Autodesk Fusion 360 part; units mm, degrees
sketch "Sketch1" plane through (0, 0, 0) normal (0, 1, 0) x (1, 0, 0)
  circle A0 centre (0, 0) radius 5.5
  dimension "d1" = 11
ref_plane "WorkPlane1" through (0, 20, 0) normal (0, 1, 0) x (1, 0, 0)
sketch "Sketch2" plane through (0, 20, 0) normal (0, 1, 0) x (1, 0, 0)
  circle A0 centre (0, 0) radius 5.5
  dimension "d3" = 11
ref_plane "WorkPlane2" through (0, -2, 0) normal (0, 1, 0) x (1, 0, 0)
sketch "Sketch3" plane through (0, -2, 0) normal (0, 1, 0) x (1, 0, 0)
  circle A0 centre (0, 0) radius 4.5
  dimension "d5" = 9
ref_plane "WorkPlane3" through (0, -5, 0) normal (0, 1, 0) x (1, 0, 0)
sketch "Sketch4" plane through (0, -5, 0) normal (0, 1, 0) x (1, 0, 0)
  circle A0 centre (0, 0) radius 4.5
  dimension "d7" = 9
ref_plane "WorkPlane4" through (0, -16, 0) normal (0, 1, 0) x (1, 0, 0)
sketch "Sketch5" plane through (0, -16, 0) normal (0, 1, 0) x (1, 0, 0)
  circle A0 centre (0, 0) radius 3.5
  dimension "d9" = 7
loft "Loft1" add profiles "Sketch2", "Sketch1" section 1 section 2 makes body 1
loft "Loft2" add profiles "Sketch3" section 1 face at (-1.4907, 0, -0.2732) section 2 on bodies 1 bodies 1
loft "Loft3" add profiles "Sketch4" section 1 face at (0.9352, -2, -1.1727) section 2 on bodies 1 bodies 1
loft "Loft4" add profiles "Sketch5" section 1 face at (0.9352, -5, -1.1727) section 2 on bodies 1 bodies 1
sketch "Sketch6" plane through (0, 0, 0) normal (1, 0, 0) x (0, 1, 0)
  line L0 (-10.5, 5.5424) -> (-10.5, -7.5313)
  line L1 (-5, 0.5) -> (-16, 0.5)
  line L2 (-16, 0.5) -> (-16, -0.5)
  line L3 (-16, -0.5) -> (-5, -0.5)
  line L4 (-5, -0.5) -> (-5, 0.5)
  line L5 (-5, 0.5) -> (-16, -0.5) construction
  line L6 (-16, 0.5) -> (-5, -0.5) construction
  line L7 (-14, 5) -> (-13, 5)
  line L8 (-13, 5) -> (-13, -5)
  line L9 (-13, -5) -> (-14, -5)
  line L10 (-14, -5) -> (-14, 5)
  line L11 (-11, 5) -> (-10, 5)
  line L12 (-10, 5) -> (-10, -5)
  line L13 (-10, -5) -> (-11, -5)
  line L14 (-11, -5) -> (-11, 5)
  line L15 (-8, 5) -> (-7, 5)
  line L16 (-7, 5) -> (-7, -5)
  line L17 (-7, -5) -> (-8, -5)
  line L18 (-8, -5) -> (-8, 5)
  point P0 (-10.5, 0)
  point P1 (-10.5, 0)
  dimension "d10" = 11
  dimension "d11" = 1
extrude "Extrude1" cut sketch "Sketch6" along normal blind 5 and the other way blind 5 contours L0 L1 L11 L12 | L0 L1 L11 L14 | L0 L3 L12 L13 | L0 L3 L13 L14 | L1 L15 L16 L18 | L1 L7 L8 L10 | L3 L8 L9 L10 | L3 L16 L17 L18 bodies 1
sketch "Sketch7" plane through (0, -16, 0) normal (0, -1, 0) x (1, 0, 0)
  circle A0 centre (0, 0) radius 3.5
  circle A1 centre (0, 0) radius 1.75
  dimension "d16" = 3.5
extrude "Extrude2" add sketch "Sketch7" against normal blind 11 contours A1 bodies 1
sketch "Sketch8" plane through (0, 20, 0) normal (0, 1, 0) x (-1, 0, 0)
  circle A0 centre (0, 0) radius 5.5
  circle A1 centre (0, 0) radius 4
  dimension "d19" = 8
extrude "Extrude3" cut sketch "Sketch8" against normal blind 1 contours A1 bodies 1
sketch "Sketch9" plane through (0, 19, 0) normal (0, 1, 0) x (-1, 0, 0)
  circle A0 centre (0, 0) radius 4
  circle A1 centre (0, 0) radius 3
  circle A2 centre (0, 0) radius 3.4
  dimension "d22" = 6
  dimension "d23" = 6.8
extrude "Extrude4" cut sketch "Sketch9" against normal blind 10 bodies 1
sketch "Sketch10" plane through (0, 9, 0) normal (0, 1, 0) x (-1, 0, 0)
  circle A0 centre (0, 0) radius 3
  circle A1 centre (0, 0) radius 1
  dimension "d26" = 2
extrude "Extrude5" add sketch "Sketch10" along normal blind 9 contours A1 bodies 1
fillet "Fillet1" radius 0.8 1 edges at (0.9323, 18, -0.3616) on bodies 1
extrude "Extrude6" add sketch "Sketch7" along normal blind 10 contours A1 bodies 1
copy_body "Body->Comp1" bodies 1 removing the originals makes body 2 in component "Component"
sketch "Sketch11" plane through (0, 0, 0) normal (0, 0, 1) x (1, 0, 0)
  line L0 (10, 20) -> (43, 20)
  line L1 (43, 20) -> (43, -16)
  line L2 (43, -16) -> (10, -16)
  line L3 (10, -16) -> (10, 20)
component "Component" placed x (1, 0, 0) y (0, 1, 0) z (0, 0, 1) at (0, 0, 0)
Can you work these out from the model? Positions are in its coordinate system, mm. A direction names the side the tool comes from. Give positions to 0.01 mm unless a question says otherwise; leave off trailing zeros. Order: outer loops, then holes, each group sorted by start corner. A loop starts at its lowest first (then second) coordinate and runs counter-clockwise, first axis right, second up. Notation, with made-up numbers: M 13,-23.75 L 54,-23.75 A17 cw 54,5.25 Z; hole C -39.5,13.25 d7. An arc over 180 degrees is marked long. Use a Markdown table: item, result. Add a question column.
Item 1: Will these pins go through, and if not, where does the flat tip stop? pin 1 (0.5 mm diameter, centred on x = 3, y = -10.5, fed in from -Z); pin 2 (3 mm diameter, centred on x = 0.5, z = 3, fed in from -Y); pin 3 (3 mm diameter, centred on x = 0.5, y = -9.5, fed in from +Z); pin 4 (3 mm diameter, centred on x = -1, z = -1, fed in from +Y).
Item 2: We'd pull the mould along X, two halves only. Please class faces 1 (the flat face through (0, -14, -2)), 2 (the cylindrical face through (0.867, 14.577, -3.905)), 3 (the conical face through (-3.89, -11.65, -0.17)): +X half, -X half, draft (parallel to the pull), parting line (faces both ways), or undercut.
Item 3: For faces 4 (the flat face through (-2, -16, -1)), 5 (the cylindrical face through (3, 14, 0)), 6 (the flat face through (0, -7, -2)), 7 (the flat face through (3, -7.5, 0.5)), which set-ups out of +Z, -Z, +X, -X, +Y, -Y let a thin tool reach every point of the face, with its end or its side?
Item 4: If I drill on L1, parallel to Z at x = 0, y = 11; L2, parallel to Y at x = 1.5, z = 1; L3, parallel to Y at x = 1.25, z = 3.5, over which ranges is the centre line in solid material (lowest first)? Write a range as [from, to].
Item 5: Suppose I cut it at A-A (y = 1.5). List the corners of the cut face in (x, z) for me.
Item 6: Suppose I cut it at B-B (y = -12.5). List the corners of the cut face in (x, z) for me.
Answer sheet:
| question | item | result |
|---|---|---|
| 1 | pin 1 | stops at z = -0.5 |
| 1 | pin 2 | stops at y = -26 |
| 1 | pin 3 | stops at z = 4.22 |
| 1 | pin 4 | stops at y = 18 |
| 2 | face 1 | draft |
| 2 | face 2 | undercut |
| 2 | face 3 | parting line |
| 3 | face 4 | -Y |
| 3 | face 5 | +Y |
| 3 | face 6 | -Z |
| 3 | face 7 | +Z, +X |
| 4 | L1 | z = [-5.5, -4], [-3.4, -3], [-1, 1], [3, 3.4], [4, 5.5] |
| 4 | L2 | y = [-16, -14], [-13, -11], [-10, -8], [-7, 9] |
| 4 | L3 | y = [-13, -11], [-10, -8], [-7, 9] |
| 5 | outline | C 0,0 d11 |
| 6 | outline | C 0,0 d7.64 |
